from build123d import *

# Parameters (mm, degrees)
F2_ANGLE       = 180
F4_D           = 12
F4_CBORE_D     = 18
F4_CBORE_DEPTH = 20


with BuildPart() as f2:
    # F0 (on Top) → F2 (revolve, symmetric)
    with BuildSketch(Plane.XY) as f2_sk:
        Polygon((-188.75, 0), (-123, 0), (-123, 465), (-188.75, 199.4), align=None)
    revolve(axis=Axis((0, 70.437513, 0), (0, 1, 0)), revolution_arc=F2_ANGLE / 2)
    revolve(f2_sk.sketch, axis=Axis((0, 70.437513, 0), (0, -1, 0)), revolution_arc=F2_ANGLE / 2)

    # F4 (through all)
    with Locations(Plane.YZ):
        with Locations((155, 152.75), (300, 152.75), (300, -152.75), (155, -152.75)):
            CounterBoreHole(F4_D / 2, F4_CBORE_D / 2, F4_CBORE_DEPTH)


solid = f2.part
Geometry check sheet. Reference: the model listing, model coordinates, mm. A direction names the side the tool comes from. Round coordinates to 2 decimals unless told otherwise and drop trailing zeros. Loops run counter-clockwise (first coordinate to the right, second up) from the corner with the lowest first, then second, coordinate; pieces in that order, holes last.
Item 1: Access from +Z, -Z, +X, -X, +Y, -Y to the whole of each face (thin tool, end or side, straight path). Record for faces 5 (the flat face through (0, 184, 149)), 6 (the flat face through (-20, 301.9, 146.9)).
Item 2: Gauge pin test, flat ends, axial feed: pin 1 (9.5 mm diameter, centred on y = 300, z = -152.75, fed in from -X); pin 2 (5 mm diameter, centred on y = 53.5, z = 28.5, fed in from +X); pin 3 (20.5 mm diameter, centred on y = 155, z = -152.75, fed in from -X); pin 4 (2 mm diameter, centred on x = -122.5, y = 412, fed in from -Z). Record the tip position at first contact, or that the pin passes through.
Item 3: Cross-section at A-A on y = 155. Record the boundary of the cut face in (x, z).
Item 4: Cross-section at B-B on x = -50. Count the separate pieces of the cut face and the enclosed holes in it, then the cut area to 3 significant figures.
Item 5: Mould release check, pull along Z, two halves, no side actions. Record for faces 1 (the flat face through (-135, 0, -3)), 2 (the cylindrical face through (-9.86, 153.828, -143.827)), 3 (the conical face through (-156.297, 330.341, 3.438)), 4 (the cylindrical face through (-70.044, 156.301, 146.893)): pulls with the +Z half, pulls with the -Z half, needs draft (parallel to the pull), parting line crosses it, or undercut.
Item 6: Cross-section at C-C on y = 102.5. Record the boundary of the cut face in (x, z), then the cut area to 3 significant figures.
Item 7: Thickness scan on line 1 (Z direction, x = -44, y = 155); line 2 (Z direction, x = -8.25, y = 300); line 3 (Z direction, x = -50, y = 45.5). Record the ranges inside material, lowest first.
Answer sheet:
1. face 5: +Z, -Z, +X, +Y, -Y
1. face 6: +X
2. pin 1: passes through
2. pin 2: stops at x = -119.03
2. pin 3: stops at x = -123.78
2. pin 4: stops at z = -61.45
3. outline: (-118.71, -146.75) - (-20, -146.75) - (-20, -143.75) - (0, -143.75) - (0, -123) arc R123 cw to (0, 123) - (0, 143.75) - (-20, 143.75) - (-20, 146.75) - (-118.71, 146.75) arc R188.75 ccw to start; (-102.1, -158.75) arc R188.75 ccw to (0, -188.75) - (0, -161.75) - (-20, -161.75) - (-20, -158.75) - close; (-102.1, 158.75) - (-20, 158.75) - (-20, 161.75) - (0, 161.75) - (0, 188.75) arc R188.75 ccw to start
4. separate pieces: 2
4. enclosed holes: 2
4. area: 46,000 mm2
5. face 1: needs draft
5. face 2: undercut
5. face 3: parting line crosses it
5. face 4: undercut
6. outline: (0, -188.75) - (0, -123) arc R123 cw to (0, 123) - (0, 188.75) arc R188.75 ccw to start
6. area: 32,200 mm2
7. line 1: z = -183.55 to -158.75, -146.75 to -114.86, 114.86 to 146.75, 158.75 to 183.55
7. line 2: z = -163.64 to -161.75, -143.75 to -122.72, 122.72 to 143.75, 161.75 to 163.64
7. line 3: z = -182.01 to -112.38, 112.38 to 182.01
